Geometry check sheet. Reference: the model listing, model coordinates, mm. Face numbers are marked on the shaded views. Coordinates: 2 decimals unless noted, no trailing zeros. Order: outer loops, then holes, each group sorted by start corner. A loop starts at its lowest first (then second) coordinate and runs counter-clockwise, first axis right, second up. Notation, with made-up numbers: M -25.5,6.25 L 11.5,6.25 A24 ccw 11.5,34.25 Z; hole C 34.25,50 d11. An arc over 180 degrees is marked long. One line per item, written item: value. Start each with the question number.
1) Sectioned sample at C-C, the plane x = 90. Enter the section's corners in (y, z).
2) Go/stop test with flat-tipped pins: P1, Ø2, axis at x = -19.5, y = 62, coming from the -Z side; P2, Ø4, axis at x = 37, y = 66.5, coming from the +Z side; P3, Ø2.5, axis at y = 94.5, z = 4.5, coming from the -X side; P4, Ø5, axis at y = 95.5, z = 5, coming from the +X side. Record where each tip stops, or that it passes through.
3) Draft check along X on the marked faces 1 and 2. Enter one of: pulls with the +X half, pulls with the -X half, needs draft (parallel to the pull), parting line crosses it, or undercut.
4) Thickness scan on L1, parallel to Y at x = 23.5, z = 7.75; L2, parallel to Y at x = -63, z = 2; L3, parallel to Z at x = -25, y = 76. Record the ranges inside material, lowest first. Write a range as from..to.
5) Sectioned sample at B-B, the plane y = 38.5. Enter the section's corners in (x, z), then the cut area to 3 significant figures.
6) Sectioned sample at A-A, the plane z = 1.5. Enter the section's corners in (x, y), then the cut area to 3 significant figures.
```python
from build123d import *

# Parameters (mm, degrees)
SKETCH2_W           = 237.244602054
SKETCH2_H           = 68.264985558
BOSS_EXTRUDE1_DEPTH = 3
BOSS_EXTRUDE2_DEPTH = 9
SKETCH3_W           = 74.150238013
SKETCH3_H           = 9
BOSS_EXTRUDE4_DEPTH = 19
FILLET1_R           = 5


with BuildPart() as part:
    # Sketch2 → Boss-Extrude1 (new body)
    with BuildSketch(Plane.XY):
        with Locations((3.706779661, 48.692372881)):
            Rectangle(SKETCH2_W, SKETCH2_H)
        Polygon((-114.915521366, 82.82486566), (122.329080688, 82.82486566), (125.206779661, 85.942372881), (-117.793220339, 85.942372881), align=None)
        Polygon((122.329080688, 82.82486566), (122.329080688, 14.559880102), (125.206779661, 11.442372881), (125.206779661, 85.942372881), align=None)
        Polygon((122.329080688, 14.559880102), (125.206779661, 11.442372881), (-117.793220339, 11.442372881), (-117.793220339, 85.942372881), (-114.915521366, 82.82486566), (-114.915521366, 14.559880102), align=None)
    extrude(amount=BOSS_EXTRUDE1_DEPTH)

    # Sketch2_3 → Boss-Extrude2 (add)
    with BuildSketch(Plane.XY):
        Polygon((-114.915521366, 82.82486566), (122.329080688, 82.82486566), (125.206779661, 85.942372881), (-117.793220339, 85.942372881), align=None)
        Polygon((122.329080688, 82.82486566), (122.329080688, 14.559880102), (125.206779661, 11.442372881), (125.206779661, 85.942372881), align=None)
        Polygon((122.329080688, 14.559880102), (125.206779661, 11.442372881), (-117.793220339, 11.442372881), (-117.793220339, 85.942372881), (-114.915521366, 82.82486566), (-114.915521366, 14.559880102), align=None)
    extrude(amount=BOSS_EXTRUDE2_DEPTH)

    # Sketch3 → Boss-Extrude4 (add)
    with BuildSketch(Plane(origin=(0, 85.942372881, 0), x_dir=(1, 0, 0), z_dir=(0, 1, 0))):
        with Locations((7.559560342, -4.5)):
            Rectangle(SKETCH3_W, SKETCH3_H)
    extrude(amount=BOSS_EXTRUDE4_DEPTH)

    # Fillet1
    fillet1_edges = [part.edges().sort_by_distance(p)[0] for p in [
        (3.706779661, 82.82486566, 3),
        (122.329080688, 48.692372881, 3),
        (-114.915521366, 82.82486566, 6),
        (122.329080688, 82.82486566, 6),
        (122.329080688, 14.559880102, 6),
        (3.706779661, 14.559880102, 3),
        (-114.915521366, 14.559880102, 6),
        (-114.915521366, 48.692372881, 3),
        (-29.515558665, 85.942372881, 4.5),
        (44.634679348, 85.942372881, 4.5),
        (-29.515558665, 104.942372881, 4.5),
        (44.634679348, 104.942372881, 4.5),
        (125.206779661, 11.442372881, 4.5),
        (-117.793220339, 11.442372881, 4.5),
        (-117.793220339, 85.942372881, 4.5),
        (125.206779661, 85.942372881, 4.5),
    ]]
    fillet(fillet1_edges, radius=FILLET1_R)


solid = part.part
```
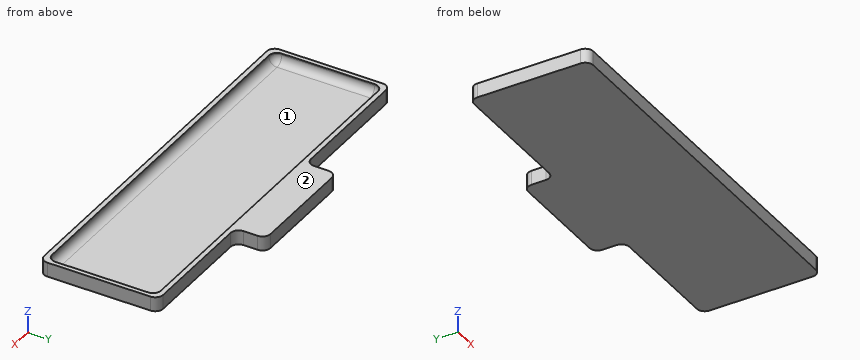
Final values:
1. outline: M 11.44,0 L 85.94,0 L 85.94,9 L 82.82,9 L 82.82,8 A5 cw 77.82,3 L 19.56,3 A5 cw 14.56,8 L 14.56,9 L 11.44,9 Z
2. P1: stops at z = 0
2. P2: stops at z = 3
2. P3: stops at x = -29.52
2. P4: stops at x = 44.63
3. face 1: undercut
3. face 2: needs draft
4. L1: y = 11.44..14.57, 82.82..104.94
4. L2: y = 11.44..85.94
4. L3: z = 0..3
5. outline: M -117.79,0 L 125.21,0 L 125.21,9 L 122.33,9 L 122.33,8 A5 cw 117.33,3 L -109.92,3 A5 cw -114.92,8 L -114.92,9 L -117.79,9 Z
5. area: 774 mm^2
6. outline: M -117.79,16.44 A5 ccw -112.79,11.44 L 120.21,11.44 A5 ccw 125.21,16.44 L 125.21,80.94 A5 ccw 120.21,85.94 L 49.63,85.94 A5 cw 44.63,90.94 L 44.63,99.94 A5 ccw 39.63,104.94 L -24.52,104.94 A5 ccw -29.52,99.94 L -29.52,90.94 A5 cw -34.52,85.94 L -112.79,85.94 A5 ccw -117.79,80.94 Z
6. area: 19,500 mm^2
